```python
from build123d import *

# Parameters (mm, degrees)
SKETCH1_W                                        = 152.4
SKETCH1_H                                        = 76.2
BOSS_EXTRUDE1_DEPTH                              = 25.4
HOLE1_D                                          = 9.525
HOLE1_CBORE_D                                    = 12.7
HOLE1_CBORE_DEPTH                                = 1.5875
F_1_2_0_5_DIAMETER_HOLE1_D                       = 12.7
CBORE_FOR_1_4_SOCKET_HEAD_CAP_SCREW1_D           = 6.7564
CBORE_FOR_1_4_SOCKET_HEAD_CAP_SCREW1_CBORE_D     = 11.1125
CBORE_FOR_1_4_SOCKET_HEAD_CAP_SCREW1_CBORE_DEPTH = 6.35
CUT_EXTRUDE2_DEPTH                               = 12.7
SKETCH22_W                                       = 0.8255
SKETCH22_H                                       = 29.718728574
CUT_EXTRUDE4_DEPTH                               = 108.010322277


with BuildPart() as part:
    # Sketch1 → Boss-Extrude1 (new body)
    with BuildSketch(Plane.XY):
        with Locations((0.410445336, 32.162996942)):
            Rectangle(SKETCH1_W, SKETCH1_H)
    extrude(amount=BOSS_EXTRUDE1_DEPTH)

    # Hole1 (through all)
    with Locations(Plane.XY.offset(25.4)):
        with Locations((0.410445336, 32.162996942)):
            CounterBoreHole(HOLE1_D / 2, HOLE1_CBORE_D / 2, HOLE1_CBORE_DEPTH)

    # 1/2 (0.5) Diameter Hole1 (through all)
    with Locations(Plane.XY.offset(25.4)):
        with Locations((-50.389554664, 34.207696942)):
            Hole(F_1_2_0_5_DIAMETER_HOLE1_D / 2)

    # CBORE for 1/4 Socket Head Cap Screw1 (through all)
    with Locations(Plane.XY.offset(25.4)):
        with Locations((-31.339554664, 63.912996942), (-31.339554664, 0.412996942), (32.160445336, 0.412996942), (32.160445336, 63.912996942)):
            CounterBoreHole(CBORE_FOR_1_4_SOCKET_HEAD_CAP_SCREW1_D / 2, CBORE_FOR_1_4_SOCKET_HEAD_CAP_SCREW1_CBORE_D / 2, CBORE_FOR_1_4_SOCKET_HEAD_CAP_SCREW1_CBORE_DEPTH)

    # Sketch14 → Cut-Extrude2 (cut)
    with BuildSketch(Plane(origin=(0, 0, 0), x_dir=(-1, 0, 0), z_dir=(0, 0, -1))):
        with BuildLine():
            Line((-13.110445336, 32.162996942), (-13.110445336, -5.937003058))
            Line((-13.110445336, -5.937003058), (12.289554664, -5.937003058))
            Line((12.289554664, -5.937003058), (12.289554664, 32.162996942))
            ThreePointArc((12.289554664, 32.162996942), (-0.410445336, 44.862996942), (-13.110445336, 32.162996942))
        make_face()
    extrude(amount=-CUT_EXTRUDE2_DEPTH, mode=Mode.SUBTRACT)

    # Sketch22 → Cut-Extrude4 (cut, through all)
    with BuildSketch(Plane.XY.offset(25.4)):
        with Locations((-50.389554664, 55.403632655)):
            Rectangle(SKETCH22_W, SKETCH22_H)
    extrude(amount=-CUT_EXTRUDE4_DEPTH, mode=Mode.SUBTRACT)


solid = part.part
```
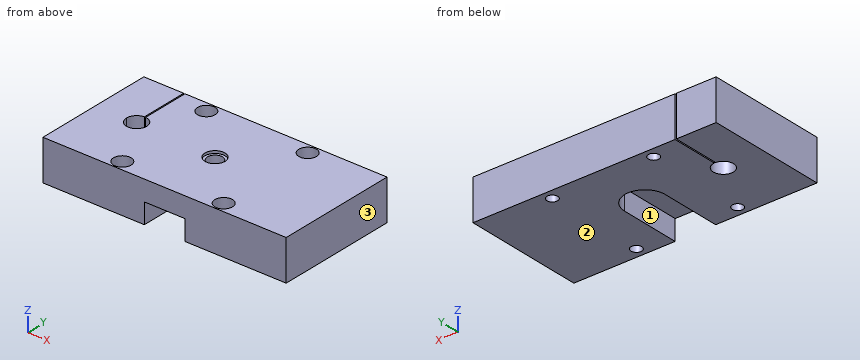
Read the model definition and answer for the solid it produces. Units are mm, in the model's axes. Face numbers are marked on the shaded views. Give positions to 0.01 mm unless a question says otherwise; leave off trailing zeros. Order: outer loops, then holes, each group sorted by start corner. A loop starts at its lowest first (then second) coordinate and runs counter-clockwise, first axis right, second up.
(1) Find section A-A (z = 3.5). Give the vertices of the cut face in (x, y), plus the area to 3 significant figures.
(2) Find section C-C (x = 3). Give the vertices of the cut face in (y, z) (1 decimal), plus the area to 3 significant figures.
(3) Straight lines are drawn through the part: L1, parallel to X at y = 9, z = 9.5; L2, parallel to X at y = 49.5, z = 16; L3, parallel to Y at x = 28, z = 19.5. For each, find the intervals that lie inside material, in ascending order.
(4) For a pull along X with two mould halves and no side action, classify the marked faces 1, 2 and 3 as released by +X, released by -X, zero draft, split by the parting line, or undercut.
(5) Given pin 1 (3.5 mm diameter, centred on x = 31, y = 66, fed in from +Z); pin 2 (2 mm diameter, centred on x = -3.5, z = 9, fed in from -Y), each flat-ended and moving along its own axis, determine where each tip first touches the part or whether it passes through.
(6) Find section B-B (y = 21). Give the vertices of the cut face in (x, z).
(7) Find section D-D (z = 15.75). Give the number of separate pieces and of enclosed holes in the cut face, plus the area to 3 significant figures.
Result sheet:
1. outline: (-75.79, -5.94) - (-12.29, -5.94) - (-12.29, 32.16) arc R12.7 cw to (13.11, 32.16) - (13.11, -5.94) - (76.61, -5.94) - (76.61, 70.26) - (-49.98, 70.26) - (-49.98, 40.54) arc R6.35 cw (long way) to (-50.8, 40.54) - (-50.8, 70.26) - (-75.79, 70.26) - close; hole circle Ø6.76 at (-31.34, 0.41); hole circle Ø6.76 at (-31.34, 63.91); hole circle Ø6.76 at (32.16, 0.41); hole circle Ø6.76 at (32.16, 63.91)
1. area: 10,100 mm2
2. outline: (-5.9, 12.7) - (28.2, 12.7) - (28.2, 23.8) - (26.4, 23.8) - (26.4, 25.4) - (-5.9, 25.4) - close; (36.2, 12.7) - (44.6, 12.7) - (44.6, 0) - (70.3, 0) - (70.3, 25.4) - (38, 25.4) - (38, 23.8) - (36.2, 23.8) - close
2. area: 1,190 mm2
3. L1: x = -75.79 to -12.29, 13.11 to 76.61
3. L2: x = -75.79 to -50.8, -49.98 to 76.61
3. L3: y = -5.94 to -3.27, 4.1 to 60.23, 67.6 to 70.26
4. face 1: undercut
4. face 2: zero draft
4. face 3: released by +X
5. pin 1: stops at z = 19.05
5. pin 2: stops at y = 43.88
6. outline: (-75.79, 0) - (-12.29, 0) - (-12.29, 12.7) - (13.11, 12.7) - (13.11, 0) - (76.61, 0) - (76.61, 25.4) - (-75.79, 25.4) - close
7. separate pieces: 1
7. enclosed holes: 5
7. area: 11,200 mm2
